For this review, take the finished solid that the model builds, in its own axes (mm). A direction names the side the tool comes from. Round coordinates to 2 decimals unless told otherwise and drop trailing zeros. Write each loop counter-clockwise with the first axis right and the second up, starting at its lowest first coordinate (ties: lowest second). Pieces come first, ordered by that corner, then holes. Notation, with made-up numbers: M -38,52.25 L 17,52.25 A22 ccw 17,65.25 Z; hole C -36,33.25 d4. An arc over 180 degrees is marked long. Use one line per item in the form item = value. Start each with the question number.
Item 1: For P1, Ø3.5, axis at x = -69, y = -47, coming from the +Z side; P2, Ø2, axis at y = -7, z = 32, coming from the -X side; P3, Ø1, axis at x = -53.5, z = 39.5, coming from the +Y side, all flat-tipped, find the tip position at first contact; note any pin that passes through.
Item 2: Add section B-B (x = -57). State the section outline as (y, z) points.
Item 3: Add section D-D (y = -39). State the section outline as (x, z) points, and give its area (3 significant figures).
Item 4: Add section A-A (y = -8). State the section outline as (x, z) points, and give its area (3 significant figures).
Item 5: For line 1 (Z direction, x = -50.5, y = -21); line 2 (Z direction, x = -69.5, y = -24); line 3 (Y direction, x = -68.5, z = 39), list the stretches that pass through material, from the lowest coordinate up. Write a range as [from, to].
Item 6: Draft analysis for pull direction Y (two halves, no side actions). For faces 1 (the flat face through (-62.926, 7.814, 29.343)), 2 (the flat face through (-61.52, -35.284, 30.361)), 3 (the flat face through (-76.73, 6.3, 36.2)), state which applies: released by +Y, released by -Y, zero draft, split by the parting line, or undercut.
Item 7: For faces 4 (the flat face through (-62, -49.838, 2)), 5 (the flat face through (-56.2, -31.838, 2.7)), 6 (the cylindrical face through (-49.77, -24.79, 54.34)), 7 (the flat face through (-62, -46, 3)), 8 (the flat face through (-63, -36, 3)), list the 3-axis set-ups (+Z, -Z, +X, -X, +Y, -Y) from which the entire face can be reached by the end or side of a thin tool; tool diameter is ignored.
Item 8: Add section C-C (z = 37.5). State the section outline as (x, y) points, and give its area (3 significant figures).
from build123d import *

# Parameters (mm, degrees)
BOSS_EXTRU_1_DEPTH      = 30
CONG_5_R                = 3.5
ESQUISSE3_R             = 1.5
ENL_V_MAT_EXTRU_1_DEPTH = 108.552111318
COQUE5_START            = -74.72972973
COQUE5_DEPTH            = 26
BOSS_EXTRU_5_DEPTH      = 4
BOSS_EXTRU_6_START      = 4
BOSS_EXTRU_6_DEPTH      = 4
ENL_V_START             = -2
ENL_V_MAT_EXTRU_5_DEPTH = 2
ESQUISSE11_W            = 30
ESQUISSE11_H            = 3
BOSS_EXTRU_8_DEPTH      = 18
NERVURE1_REACH          = 85.236
ESQUISSE12_WALL_W       = 25.034902344
ESQUISSE12_WALL_H       = 2
ESQUISSE13_R            = 0.75
ENL_V_MAT_EXTRU_6_DEPTH = 8
BOSS_EXTRU_9_DEPTH      = 6
BOSS_EXTRU_10_DEPTH     = 2.5
CONG_7_R                = 2
ENL_V_MAT_EXTRU_7_DEPTH = 4
CONG_9_R                = 5
ESQUISSE22_R            = 1.4
ENL_V_MAT_EXTRU_8_DEPTH = 108.552111389


# Read off the part's stored shape, not the designer's step: Coque5
with BuildPart() as part:
    # Esquisse2 → Boss.-Extru.1 (new body)
    with BuildSketch(Plane(origin=(-46.72972973, 0, -4), x_dir=(0, 1, 0), z_dir=(1, 0, 0))):
        Polygon((-49.837837838, 4), (-40.553869421, 4), (-32.813706623, 32.034902345), (7.138030947, 32.034902345), (14.878193746, 4), (24.162162162, 4), (24.162162162, 7), (17.162162162, 7), (1.553427739, 63.534902), (-27.229103415, 63.534902), (-42.837837838, 7), (-49.837837838, 7), align=None)
        Polygon((-31.571300562, 36.534902345), (5.895624886, 36.534902345), (-0.316405324, 59.034902), (-25.359270352, 59.034902), align=None, mode=Mode.SUBTRACT)
    extrude(amount=-BOSS_EXTRU_1_DEPTH)

    # Congé5
    cong_5_edges = [part.edges().sort_by_distance(p)[0] for p in [
        (-61.72972973, -27.229103415, 59.534902),
        (-61.72972973, 1.553427739, 59.534902),
        (-61.72972973, -25.359270352, 55.034902),
        (-61.72972973, -0.316405324, 55.034902),
    ]]
    fillet(cong_5_edges, radius=CONG_5_R)

    # Esquisse3 → Enlèv. mat.-Extru.1 (cut, through all)
    with BuildSketch(Plane.XY.offset(3)):
        with Locations((-69.22972973, 20.662162162)):
            Circle(ESQUISSE3_R)
        with Locations(Location((-54.22972973, 20.662162162, 0), (0, 0, 180))):
            Circle(ESQUISSE3_R)
        with Locations((-54.22972973, -46.337837838)):
            Circle(ESQUISSE3_R)
        with Locations(Location((-69.22972973, -46.337837838, 0), (0, 0, 180))):
            Circle(ESQUISSE3_R)
    extrude(amount=-ENL_V_MAT_EXTRU_1_DEPTH, mode=Mode.SUBTRACT)

    # Coque5 outline → Coque5 (cut)
    with BuildSketch(Plane.YZ.offset(COQUE5_START)):
        with BuildLine():
            Line((-26.010377917, 56.434102065), (-41.039101991, 2))
            Line((-41.039101991, 2), (-40.00168895, 2))
            Line((-40.00168895, 2), (-32.813706623, 28.034902345))
            Line((-32.813706623, 28.034902345), (7.138030947, 28.034902345))
            Line((7.138030947, 28.034902345), (14.326013274, 2))
            Line((14.326013274, 2), (15.363426315, 2))
            Line((15.363426315, 2), (0.334702242, 56.434102065))
            ThreePointArc((0.334702242, 56.434102065), (-0.202576772, 57.22838432), (-1.11120208, 57.534902))
            Line((-1.11120208, 57.534902), (-24.564473595, 57.534902))
            ThreePointArc((-24.564473595, 57.534902), (-25.473098904, 57.22838432), (-26.010377917, 56.434102065))
        make_face()
        with BuildLine():
            Line((-31.571300562, 32.534902345), (-26.068417283, 52.466368819))
            ThreePointArc((-26.068417283, 52.466368819), (-24.814766252, 54.319694081), (-22.694640532, 55.034902))
            Line((-22.694640532, 55.034902), (-2.981035143, 55.034902))
            ThreePointArc((-2.981035143, 55.034902), (-0.860909424, 54.319694081), (0.392741608, 52.466368819))
            Line((0.392741608, 52.466368819), (5.895624886, 32.534902345))
            Line((5.895624886, 32.534902345), (-31.571300562, 32.534902345))
        make_face(mode=Mode.SUBTRACT)
    extrude(amount=COQUE5_DEPTH, mode=Mode.SUBTRACT)

    # Esquisse6 → Boss.-Extru.5 (add)
    with BuildSketch(Plane.ZY.offset(48.72972973)):
        Polygon((32.534902345, -32.608713603), (28.034902345, -33.851119664), (28.034902345, 8.175443988), (32.534902345, 6.933037927), align=None)
    extrude(amount=BOSS_EXTRU_5_DEPTH)

    # Esquisse7 → Boss.-Extru.6 (add)
    with BuildSketch(Plane.ZY.offset(48.72972973).offset(BOSS_EXTRU_6_START)):
        with BuildLine():
            Line((57.534902, -24.564473595), (57.534902, -1.11120208))
            ThreePointArc((57.534902, -1.11120208), (57.22838432, -0.202576772), (56.434102065, 0.334702242))
            Line((56.434102065, 0.334702242), (32.534902345, 6.933037927))
            Line((32.534902345, 6.933037927), (32.534902345, 5.895624886))
            Line((32.534902345, 5.895624886), (52.466368819, 0.392741608))
            ThreePointArc((52.466368819, 0.392741608), (54.319694081, -0.860909424), (55.034902, -2.981035143))
            Line((55.034902, -2.981035143), (55.034902, -22.694640532))
            ThreePointArc((55.034902, -22.694640532), (54.319694081, -24.814766252), (52.466368819, -26.068417283))
            Line((52.466368819, -26.068417283), (32.534902345, -31.571300562))
            Line((32.534902345, -31.571300562), (32.534902345, -32.608713603))
            Line((32.534902345, -32.608713603), (56.434102065, -26.010377917))
            ThreePointArc((56.434102065, -26.010377917), (57.22838432, -25.473098904), (57.534902, -24.564473595))
        make_face()
    extrude(amount=-BOSS_EXTRU_6_DEPTH)

    # Esquisse9 → Enlèv. mat.-Extru.5 (cut)
    with BuildSketch(Plane(origin=(-74.72972973, 0, 0), x_dir=(0, 0, -1), z_dir=(1, 0, 0)).offset(ENL_V_START)):
        with BuildLine():
            Line((-2, 15.363426315), (-56.434102065, 0.334702242))
            ThreePointArc((-56.434102065, 0.334702242), (-57.22838432, -0.202576772), (-57.534902, -1.11120208))
            Line((-57.534902, -1.11120208), (-57.534902, -24.564473595))
            ThreePointArc((-57.534902, -24.564473595), (-57.22838432, -25.473098904), (-56.434102065, -26.010377917))
            Line((-56.434102065, -26.010377917), (-2, -41.039101991))
            Line((-2, -41.039101991), (-2, -40.00168895))
            Line((-2, -40.00168895), (-28.034902345, -32.813706623))
            Line((-28.034902345, -32.813706623), (-28.034902345, 7.138030947))
            Line((-28.034902345, 7.138030947), (-2, 14.326013274))
            Line((-2, 14.326013274), (-2, 15.363426315))
        make_face()
    extrude(amount=ENL_V_MAT_EXTRU_5_DEPTH, mode=Mode.SUBTRACT)

    # Esquisse11 → Boss.-Extru.8 (add)
    with BuildSketch(Plane.XZ.offset(49.837837838)):
        with Locations((-61.72972973, 1.5)):
            Rectangle(ESQUISSE11_W, ESQUISSE11_H)
    boss_extru_8 = extrude(amount=-BOSS_EXTRU_8_DEPTH)

    # Esquisse12 wall → Nervure1 (add, up to next)
    with BuildSketch(Plane(origin=(-46.72972973, -31.837837838, 15.517451172), x_dir=(0, 0, -1), z_dir=(0, 1, 0)), mode=Mode.PRIVATE) as nervure1_sk1:
        with Locations((0, 1)):
            Rectangle(ESQUISSE12_WALL_W, ESQUISSE12_WALL_H)
    nervure1_tool1 = extrude(nervure1_sk1.sketch, amount=-NERVURE1_REACH, mode=Mode.PRIVATE) - part.part
    nervure1 = nervure1_tool1.solids().sort_by_distance((-46.72972973, -31.837837838, 15.517451172))[0]
    add(nervure1)

    # Symétrie1: Boss.-Extru.8, Nervure1 across plane
    add(boss_extru_8.mirror(Plane.ZX.offset(-12.837837838)))
    add(nervure1.mirror(Plane.ZX.offset(-12.837837838)))

    # Esquisse13 → Enlèv. mat.-Extru.6 (cut)
    with BuildSketch(Plane(origin=(-46.72972973, 0, 0), x_dir=(0, 0, -1), z_dir=(1, 0, 0))):
        with Locations((-57.618809014, -12.837837838)):
            Circle(ESQUISSE13_R)
        with Locations((-29.818809014, -12.837837838)):
            Circle(ESQUISSE13_R)
    extrude(amount=-ENL_V_MAT_EXTRU_6_DEPTH, mode=Mode.SUBTRACT)

    # Esquisse15 → Boss.-Extru.9 (add)
    with BuildSketch(Plane.ZY.offset(52.72972973)):
        with BuildLine():
            Line((57.534902, -15.386456996), (57.534902, -13.583129467))
            ThreePointArc((57.534902, -13.583129467), (56.868809014, -12.837837838), (57.534902, -12.092546208))
            Line((57.534902, -12.092546208), (57.534902, -10.28921868))
            ThreePointArc((57.534902, -10.28921868), (55.068809014, -12.837837838), (57.534902, -15.386456996))
        make_face()
    extrude(amount=BOSS_EXTRU_9_DEPTH)

    # Esquisse16 → Boss.-Extru.10 (add)
    with BuildSketch(Plane.ZY.offset(58.72972973)):
        with BuildLine():
            Line((57.534902, -15.386456996), (57.534902, -10.28921868))
            ThreePointArc((57.534902, -10.28921868), (55.068809014, -12.837837838), (57.534902, -15.386456996))
        make_face()
    extrude(amount=BOSS_EXTRU_10_DEPTH)

    # Congé7
    cong_7_edges = [part.edges().sort_by_distance(p)[0] for p in [
        (-61.22972973, -12.837837838, 55.068809014),
    ]]
    fillet(cong_7_edges, radius=CONG_7_R)

    # Esquisse17 → Enlèv. mat.-Extru.7 (cut)
    with BuildSketch(Plane.ZY.offset(52.72972973)):
        with BuildLine():
            Line((30.034902345, 6.585850475), (32.534902345, 5.895624886))
            Line((32.534902345, 5.895624886), (32.534902345, -31.571300562))
            Line((32.534902345, -31.571300562), (30.034902345, -32.261526151))
            Line((30.034902345, -32.261526151), (30.034902345, -15.378665198))
            ThreePointArc((30.034902345, -15.378665198), (32.368809014, -12.837837838), (30.034902345, -10.297010478))
            Line((30.034902345, -10.297010478), (30.034902345, 6.585850475))
        make_face()
    extrude(amount=-ENL_V_MAT_EXTRU_7_DEPTH, mode=Mode.SUBTRACT)

    # Congé9
    cong_9_edges = [part.edges().sort_by_distance(p)[0] for p in [
        (-76.72972973, -49.837837838, 1.5),
        (-76.72972973, 24.162162162, 1.5),
        (-46.72972973, 24.162162162, 1.5),
        (-46.72972973, -49.837837838, 1.5),
    ]]
    fillet(cong_9_edges, radius=CONG_9_R)

    # Esquisse22 → Enlèv. mat.-Extru.8 (cut, through all)
    with BuildSketch(Plane.XY.offset(3)):
        with Locations((-69.114577733, 20.662162162)):
            Circle(ESQUISSE22_R)
        with Locations(Location((-54.344881726, 20.662162162, 0), (0, 0, 180))):
            Circle(ESQUISSE22_R)
        with Locations((-54.344881726, -46.337837838)):
            Circle(ESQUISSE22_R)
        with Locations(Location((-69.114577733, -46.337837838, 0), (0, 0, 180))):
            Circle(ESQUISSE22_R)
    extrude(amount=-ENL_V_MAT_EXTRU_8_DEPTH, mode=Mode.SUBTRACT)


solid = part.part
Calculated:
q1.P1 = 3
q1.P2 = -48.73
q1.P3 = 7.22
q2.outline = M -49.84,0 L -31.84,0 L -31.84,3 L -40.76,3 L -26.01,56.43 A1.5 cw -24.56,57.53 L -15.39,57.53 A2.55 ccw -10.29,57.53 L -1.11,57.53 A1.5 cw 0.33,56.43 L 15.09,3 L 6.16,3 L 6.16,0 L 24.16,0 L 24.16,3 L 17.16,3 L 2.26,56.97 A3.5 ccw -1.11,59.53 L -24.56,59.53 A3.5 ccw -27.94,56.97 L -42.84,3 L -49.84,3 Z; hole M -13.58,57.53 A0.75 ccw -12.09,57.53 Z
q3.outline = M -76.73,0 L -46.73,0 L -46.73,16.9 L -76.73,16.9 L -76.73,9.39 L -48.73,9.39 L -48.73,3 L -76.73,3 Z
q3.area = 328 mm^2
q4.outline = M -76.73,57.53 L -52.73,57.53 L -52.73,55.03 L -46.73,55.03 L -46.73,59.53 L -76.73,59.53 Z; M -52.73,28.03 L -46.73,28.03 L -46.73,32.53 L -48.73,32.53 L -48.73,30.03 L -52.73,30.03 Z
q4.area = 92.0 mm^2
q5.line_1 = [28.03, 30.03], [55.03, 59.53]
q5.line_2 = [57.53, 59.53]
q5.line_3 = [-32.9, -30.82], [5.15, 7.22]
q6.face_1 = undercut
q6.face_2 = released by -Y
q6.face_3 = zero draft
q7.face_4 = +Z, -Z, +X, -X, -Y
q7.face_5 = -Z, +X, -X
q7.face_6 = +X, -X
q7.face_7 = +Z, +X, -X, -Y
q7.face_8 = -X
q8.outline = M -76.73,-33.31 L -46.73,-33.31 L -46.73,-30.2 L -52.73,-30.2 L -52.73,-31.24 L -76.73,-31.24 Z; M -76.73,5.56 L -52.73,5.56 L -52.73,4.52 L -46.73,4.52 L -46.73,7.64 L -76.73,7.64 Z
q8.area = 137 mm^2
